Design review of the part built by this model. Coordinates are the model's own, in mm. Face numbers are marked on the shaded views. A direction names the side the tool comes from. Coordinates: 2 decimals unless noted, no trailing zeros. Order: outer loops, then holes, each group sorted by start corner. A loop starts at its lowest first (then second) coordinate and runs counter-clockwise, first axis right, second up. Notation, with made-up numbers: (48, -12) -> (101, -12) arc R23 cw to (101, -2) -> close; hole circle Ø4 at (71, 9.25). An arc over 180 degrees is marked (long way). Use a Markdown table: item, result. Add a question column.
Q1. Add section A-A (y = 10). State the section outline as (x, z) points.
Q2. Machinability: for the marked faces 4 and 5, which of the approach directions +Z, -Z, +X, -X, +Y, -Y give a long, thin tool a straight path to every point of the face, cutting with its end or side? Answer none if there is none.
Q3. Add section B-B (z = 32). State the section outline as (x, y) points.
Q4. Wall thickness on probe 1 along X at (y, z) = (-14.5, 84); probe 2 along Y at (x, z) = (0, 54): over which ranges is each line inside the solid? List them lowest first.
Q5. The part is to be moulded in two halves that separate along Y. For the marked faces 1, 2 and 3, say which applies: pulls with the +Y half, pulls with the -Y half, needs draft (parallel to the pull), parting line crosses it, or undercut.
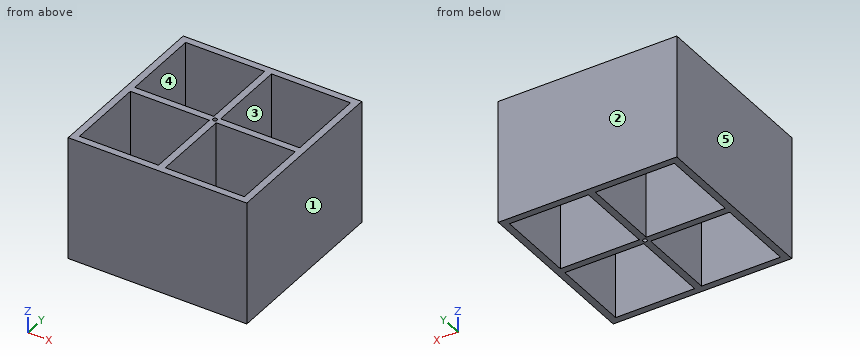
from build123d import *

# Parameters (mm, degrees)
SKICA1_W                 = 130
SKICA1_H                 = 130
P_IDAT_VYSUNUT_M1_DEPTH  = 90
SKICA3_W                 = 57.5
SKICA3_H                 = 57.5
ODEBRAT_VYSUNUT_M1_DEPTH = 90
SKICA4_R                 = 1.5
ODEBRAT_VYSUNUT_M2_DEPTH = 90


with BuildPart() as part:
    # Skica1 → Přidat vysunutím1 (new body)
    with BuildSketch(Plane.XY):
        Rectangle(SKICA1_W, SKICA1_H)
    extrude(amount=P_IDAT_VYSUNUT_M1_DEPTH)

    # Skica3 → Odebrat vysunutím1 (cut)
    with BuildSketch(Plane.XY.offset(90)):
        with Locations((-31.25, 31.25)):
            Rectangle(SKICA3_W, SKICA3_H)
        with Locations((31.25, 31.25)):
            Rectangle(SKICA3_W, SKICA3_H)
        with Locations((-31.25, -31.25)):
            Rectangle(SKICA3_W, SKICA3_H)
        with Locations((31.25, -31.25)):
            Rectangle(SKICA3_W, SKICA3_H)
    extrude(amount=-ODEBRAT_VYSUNUT_M1_DEPTH, mode=Mode.SUBTRACT)

    # Skica4 → Odebrat vysunutím2 (cut)
    with BuildSketch(Plane.XY.offset(90)):
        Circle(SKICA4_R)
    extrude(amount=-ODEBRAT_VYSUNUT_M2_DEPTH, mode=Mode.SUBTRACT)


solid = part.part
Established:
| question | item | result |
|---|---|---|
| 1 | outline | (-65, 0) -> (-60, 0) -> (-60, 90) -> (-65, 90) -> close; (-2.5, 0) -> (2.5, 0) -> (2.5, 90) -> (-2.5, 90) -> close; (60, 0) -> (65, 0) -> (65, 90) -> (60, 90) -> close |
| 2 | face 4 | +Z, -Z |
| 2 | face 5 | +Z, -Z, -X, +Y, -Y |
| 3 | outline | (-65, -65) -> (65, -65) -> (65, 65) -> (-65, 65) -> close; hole (-60, -60) -> (-2.5, -60) -> (-2.5, -2.5) -> (-60, -2.5) -> close; hole (-60, 2.5) -> (-2.5, 2.5) -> (-2.5, 60) -> (-60, 60) -> close; hole circle Ø3 at (0, 0); hole (2.5, -60) -> (60, -60) -> (60, -2.5) -> (2.5, -2.5) -> close; hole (2.5, 2.5) -> (60, 2.5) -> (60, 60) -> (2.5, 60) -> close |
| 4 | probe 1 | -65 to -60, -2.5 to 2.5, 60 to 65 |
| 4 | probe 2 | -65 to -1.5, 1.5 to 65 |
| 5 | face 1 | needs draft |
| 5 | face 2 | pulls with the +Y half |
| 5 | face 3 | undercut |
